For this review, use the dimensioned drawing (mm, ordinates from the lowest corner) and the shaded views. A direction names the side the tool comes from. Round coordinates to 2 decimals unless told otherwise and drop trailing zeros. Order: outer loops, then holes, each group sorted by start corner. A loop starts at its lowest first (then second) coordinate and runs counter-clockwise, first axis right, second up. Notation, with made-up numbers: (43, 23) - (76, 23) arc R26 ccw to (76, 45) - close; hole circle Ø6 at (-37, 34). An arc over 180 degrees is marked (long way). Write each question's results on one line, items separated by ' | '. Start each with the question number.
(1) Take a section at D-D, the plane x = 27. Give the boundary of the cut face in (y, z).
(2) Take a section at C-C, the plane y = 10.5. Give the boundary of the cut face in (x, z), plus the area to 3 significant figures.
(3) Take a section at B-B, the plane z = 40. Give the boundary of the cut face in (x, y).
(4) For L1, parallel to Z at x = 25.4, y = 22; L2, parallel to X at y = 16, z = 44; L3, parallel to Y at x = 17, z = 26.5, list the stretches that pass through material, from the lowest coordinate up. Write a range as from..to.
(5) Take a section at A-A, the plane y = 28. Give the boundary of the cut face in (x, z).
(6) Insertion check: pin 1 Ø4 at (y, z) = (23.5, 46.5) entering from +X; pin 2 Ø14 at (y, z) = (25.5, 37.5) entering from -X; pin 3 Ø10 at (y, z) = (10, 12.5) entering from +X; pin 4 Ø12 at (y, z) = (18.5, 22.5) entering from -X. Each pin has a flat end and moves straight along its axis. Give the tip position at first contact, or say it passes through.
(7) For the marked faces 4, 5 and 6, list the 3-axis set-ups (+Z, -Z, +X, -X, +Y, -Y) from which the entire face can be reached by the end or side of a thin tool; tool diameter is ignored.
(8) Draft analysis for pull direction Z (two halves, no side actions). For the marked faces 1, 2 and 3, state which applies: pulls with the +Z half, pulls with the -Z half, needs draft (parallel to the pull), parting line crosses it, or undercut.
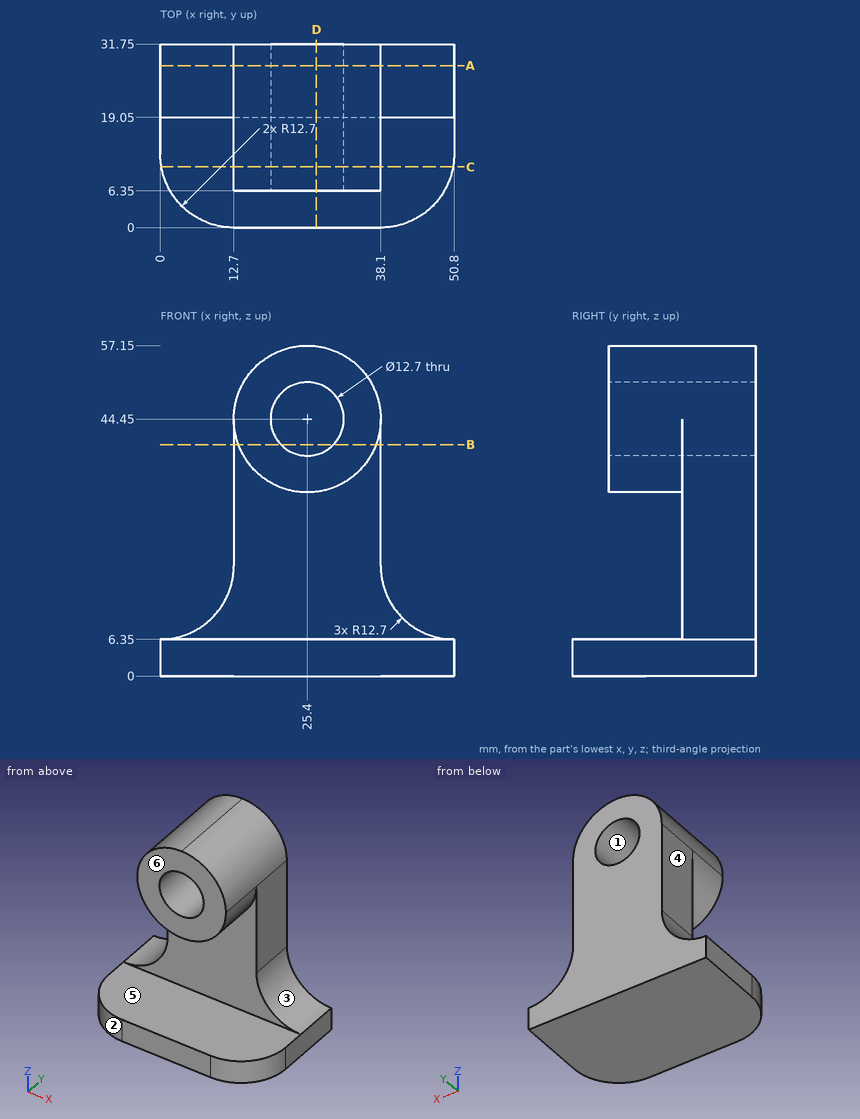
Results below:
1) outline: (0, 0) - (31.75, 0) - (31.75, 38.3) - (6.35, 38.3) - (6.35, 31.85) - (19.05, 31.85) - (19.05, 6.35) - (0, 6.35) - close; (6.35, 50.6) - (31.75, 50.6) - (31.75, 57.05) - (6.35, 57.05) - close
2) outline: (0.19, 0) - (50.61, 0) - (50.61, 6.35) - (0.19, 6.35) - close; circle Ø25.4 at (25.4, 44.45); hole circle Ø12.7 at (25.4, 44.45) | area: 700 mm^2
3) outline: (12.7, 19.05) - (13.51, 19.05) - (13.51, 6.35) - (20.87, 6.35) - (20.87, 31.75) - (12.7, 31.75) - close; (29.93, 6.35) - (37.29, 6.35) - (37.29, 19.05) - (38.1, 19.05) - (38.1, 31.75) - (29.93, 31.75) - close
4) L1: z = 0..38.1, 50.8..57.15 | L2: x = 12.71..19.07, 31.73..38.09 | L3: y = 19.05..31.75
5) outline: (0, 0) - (50.8, 0) - (50.8, 6.35) arc R12.7 cw to (38.1, 19.05) - (38.1, 44.45) arc R12.7 ccw to (12.7, 44.45) - (12.7, 19.05) arc R12.7 cw to (0, 6.35) - close; hole circle Ø12.7 at (25.4, 44.45)
6) pin 1: stops at x = 38.1 | pin 2: stops at x = 12.7 | pin 3: passes through | pin 4: stops at x = 12.45
7) face 4: +Z, -X, +Y, -Y | face 5: +X, -X, -Y | face 6: +Z, +X, -X, -Y
8) face 1: undercut | face 2: needs draft | face 3: pulls with the +Z half
